Read the model definition and answer for the solid it produces. Units are mm, in the model's axes. Round coordinates to 2 decimals unless told otherwise and drop trailing zeros. Order: outer loops, then holes, each group sorted by start corner. A loop starts at its lowest first (then second) coordinate and runs counter-clockwise, first axis right, second up. Notation, with made-up numbers: (-21, -1.5) - (26, -1.5) arc R15 cw to (26, 27.5) - close; hole circle Ø4 at (-38.75, -17.75). An arc over 180 degrees is marked (long way). One line per question, with ' | ' between items. Start each with the question number.
1) The mould has two halves that part along X. Classify faces 1 (the flat face through (8, 0, 0)), 2 (the conical face through (1.502, -0.198, -0.894)), 3 (the flat face through (0, 1, 0)), 4 (the cylindrical face through (5, 0, -1)): pulls with the +X half, pulls with the -X half, needs draft (parallel to the pull), parting line crosses it, or undercut.
2) The part is cut by section C-C, the plane z = 0. Give the vertices of the cut face in (x, y).
3) Straight lines are drawn through the part: line 1 (Z direction, x = 0.75, y = -0.75); line 2 (Z direction, x = 3.5, y = 0.85); line 3 (X direction, y = -1.1, z = 0.8). For each, find the intervals that lie inside material, in ascending order. Write a range as from..to.
4) The part is cut by section A-A, the plane y = 0. Give the vertices of the cut face in (x, z), plus the area to 3 significant figures.
5) Flat-ended cylindrical pins translate along their axes: pin 1 (1.5 mm diameter, centred on x = 4.5, z = 1, fed in from +Y); pin 2 (1 mm diameter, centred on y = -1, z = -0.5, fed in from +X); pin 3 (1.5 mm diameter, centred on x = 2.5, y = -1.5, fed in from -Z). Find the tip coordinate at first contact, or state that the pin passes through.
6) The part is cut by section B-B, the plane x = 3.25. Give the vertices of the cut face in (y, z).
from build123d import *

# Parameters (mm, degrees)
SKETCH_3_W               = 0.5
SKETCH_3_H               = 0.5
CUT_EXTRUDE_1_DEPTH      = 2.9
CUT_EXTRUDE_1_DEPTH_BACK = 2.9


with BuildPart() as part:
    # Эскиз2 → Повернуть1 (revolve)
    with BuildSketch(Plane.XY):
        with BuildLine():
            Line((0, 0), (0, 1.9))
            Line((0, 1.9), (0.2, 1.9))
            Line((0.2, 1.9), (1.126725855, 0.940347284))
            ThreePointArc((1.126725855, 0.940347284), (1.20815228, 0.889276183), (1.304000388, 0.882088693))
            Line((1.304000388, 0.882088693), (2, 1))
            Line((2, 1), (8, 1))
            Line((8, 1), (8, 0))
            Line((8, 0), (0, 0))
        make_face()
    revolve(axis=Axis((0, 0, 0), (1, 0, 0)))

    # Эскиз3 → Вырез-Вытянуть1 (cut, two sides)
    with BuildSketch(Plane.XY) as cut_extrude_1_sk:
        with Locations((0.25, 0)):
            Rectangle(SKETCH_3_W, SKETCH_3_H)
    extrude(amount=CUT_EXTRUDE_1_DEPTH, mode=Mode.SUBTRACT)
    extrude(cut_extrude_1_sk.sketch, amount=-CUT_EXTRUDE_1_DEPTH_BACK, mode=Mode.SUBTRACT)


solid = part.part
Values:
1) face 1: pulls with the +X half | face 2: undercut | face 3: pulls with the -X half | face 4: needs draft
2) outline: (0, -1.9) - (0.2, -1.9) - (1.13, -0.94) arc R0.2 cw to (1.3, -0.88) - (2, -1) - (8, -1) - (8, 1) - (2, 1) - (1.3, 0.88) arc R0.2 cw to (1.13, 0.94) - (0.2, 1.9) - (0, 1.9) - (0, 0.25) - (0.5, 0.25) - (0.5, -0.25) - (0, -0.25) - close
3) line 1: z = -1.1..1.1 | line 2: z = -0.53..0.53 | line 3: x = 0..0.72
4) outline: (0.5, -1.59) - (1.13, -0.94) arc R0.2 cw to (1.3, -0.88) - (2, -1) - (8, -1) - (8, 1) - (2, 1) - (1.3, 0.88) arc R0.2 cw to (1.13, 0.94) - (0.5, 1.59) - close | area: 15.2 mm^2
5) pin 1: stops at y = 0.97 | pin 2: stops at x = 8 | pin 3: stops at z = -0.66
6) outline: circle Ø2 at (0, 0)
